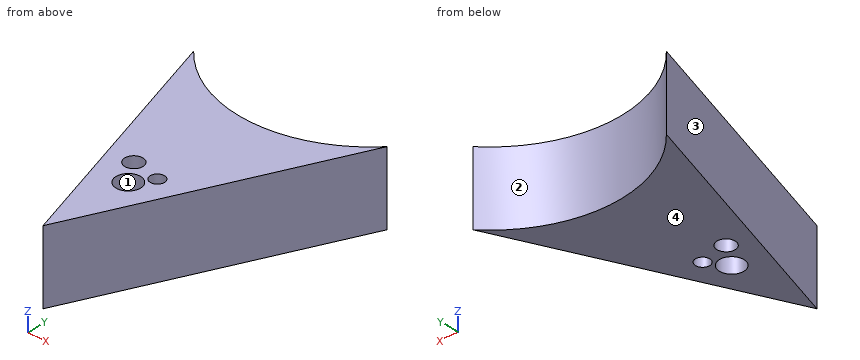
```python
from build123d import *

# Parameters (mm, degrees)
F0_R     = 4.248171
F0_R_2   = 3.148888
F0_R_3   = 2.469941
F1_DEPTH = 25.4


with BuildPart() as f1:
    # F0 (on Top) → F1 (new body)
    with BuildSketch(Plane.XY):
        with BuildLine():
            ThreePointArc((25.431026, 34.149278), (-8.564489, 18.957498), (-42.560004, 34.149278))
            Line((-42.560004, 34.149278), (-13.871806, -54.210376))
            Line((-13.871806, -54.210376), (25.431026, 34.149278))
        make_face()
        with Locations((-11.932543, -23.845781)):
            Circle(F0_R, mode=Mode.SUBTRACT)
        with Locations((-17.458783, -15.749557)):
            Circle(F0_R_2, mode=Mode.SUBTRACT)
        with Locations((-7.469992, -17.612405)):
            Circle(F0_R_3, mode=Mode.SUBTRACT)
    extrude(amount=F1_DEPTH)


solid = f1.part
```
Design review of the part built by this model. Coordinates are the model's own, in mm. Face numbers are marked on the shaded views. Give positions to 0.01 mm unless a question says otherwise; leave off trailing zeros. Order: outer loops, then holes, each group sorted by start corner. A loop starts at its lowest first (then second) coordinate and runs counter-clockwise, first axis right, second up. Notation, with made-up numbers: (62.25, 46.5) -> (90.25, 46.5) arc R20 cw to (90.25, 85.5) -> close; hole circle Ø7 at (-15, 13). An arc over 180 degrees is marked (long way). Write item = value, one per line. Start each with the question number.
(1) We need section D-D on y = -11. Write out the cut boundary in (x, z), plus the area to 3 significant figures.
(2) We need section B-B on z = 3.25. Write out the cut boundary in (x, y).
(3) Mouldability with a two-part tool opening along Y and no side actions: class the marked faces 1, 2, 3 and 4 as +Y half, -Y half, draft (parallel to the pull), parting line (faces both ways), or undercut.
(4) We need section A-A on y = -25.5. Write out the cut boundary in (x, z).
(5) For pin 1 (10 mm diameter, centred on y = 12.5, z = 6.5, fed in from +X); pin 2 (8 mm diameter, centred on x = -2.5, z = 17.5, fed in from +Y); pin 3 (12 mm diameter, centred on y = -24.5, z = 8, fed in from +X), all flat-tipped, find the tip position at first contact; note any pin that passes through.
(6) We need section C-C on x = -27.5. Write out the cut boundary in (y, z), plus the area to 3 significant figures.
(7) To check wall thickness, follow line 1 along X through (y, z) = (-16.5, 5.75); line 2 along X through (y, z) = (29.5, 6); line 3 along Y through (x, z) = (-13.5, 18.75). State the ranges of each line that lie inside material, in increasing order.
Numbers:
q1.outline = (-27.9, 0) -> (5.35, 0) -> (5.35, 25.4) -> (-27.9, 25.4) -> close
q1.area = 845 mm^2
q2.outline = (-42.56, 34.15) -> (-13.87, -54.21) -> (25.43, 34.15) arc R45.63 cw to start; hole circle Ø6.3 at (-17.46, -15.75); hole circle Ø8.5 at (-11.93, -23.85); hole circle Ø4.94 at (-7.47, -17.61)
q3.face_1 = undercut
q3.face_2 = +Y half
q3.face_3 = -Y half
q3.face_4 = draft
q4.outline = (-23.19, 0) -> (-15.85, 0) -> (-15.85, 25.4) -> (-23.19, 25.4) -> close; (-8.02, 0) -> (-1.1, 0) -> (-1.1, 25.4) -> (-8.02, 25.4) -> close
q5.pin_1 = 18.03
q5.pin_2 = 20.08
q5.pin_3 = 2.01
q6.outline = (-12.24, 0) -> (23.07, 0) -> (23.07, 25.4) -> (-12.24, 25.4) -> close
q6.area = 897 mm^2
q7.line_1 = -26.12 to -20.52, -14.4 to -9.68, -5.26 to 2.9
q7.line_2 = -41.05 to -37.74, 20.61 to 23.36
q7.line_3 = -53.37 to -27.79, -19.9 to 19.23
